from build123d import *

# Parameters (mm, degrees)
F0_R     = 4
F1_DEPTH = 3
F0_R_2   = 11
F2_DEPTH = 1


with BuildPart() as f1:
    # F0 (on Top) → F1 (new body, symmetric)
    with BuildSketch(Plane.XY):
        Circle(F0_R)
        with BuildLine():
            ThreePointArc((-2.304886, -1.5), (-2.75, 0), (-2.304886, 1.5))
            Line((-2.304886, 1.5), (2.304886, 1.5))
            ThreePointArc((2.304886, 1.5), (2.75, 0), (2.304886, -1.5))
            Line((2.304886, -1.5), (-2.304886, -1.5))
        make_face(mode=Mode.SUBTRACT)
    extrude(amount=F1_DEPTH, both=True)

    # F0 (on Top) → F2 (join, symmetric)
    with BuildSketch(Plane.XY):
        Circle(F0_R_2)
        with BuildLine():
            Line((-7.071068, -7.071068), (-4.242641, -4.242641))
            ThreePointArc((-4.242641, -4.242641), (-3.80636, -4.638063), (-3.333421, -4.988818))
            Line((-3.333421, -4.988818), (-5.555702, -8.314696))
            ThreePointArc((-5.555702, -8.314696), (-6.343933, -7.730105), (-7.071068, -7.071068))
        make_face(mode=Mode.SUBTRACT)
        with BuildLine():
            Line((-3.826834, -9.238795), (-2.296101, -5.543277))
            ThreePointArc((-2.296101, -5.543277), (-1.741708, -5.741642), (-1.170542, -5.884712))
            Line((-1.170542, -5.884712), (-1.950903, -9.807853))
            ThreePointArc((-1.950903, -9.807853), (-2.902847, -9.569403), (-3.826834, -9.238795))
        make_face(mode=Mode.SUBTRACT)
        with BuildLine():
            Line((-9.238795, -3.826834), (-5.543277, -2.296101))
            ThreePointArc((-5.543277, -2.296101), (-5.291528, -2.82838), (-4.988818, -3.333421))
            Line((-4.988818, -3.333421), (-8.314696, -5.555702))
            ThreePointArc((-8.314696, -5.555702), (-8.819213, -4.713967), (-9.238795, -3.826834))
        make_face(mode=Mode.SUBTRACT)
        with BuildLine():
            Line((-10, 0), (-6, 0))
            ThreePointArc((-6, 0), (-5.971108, -0.588103), (-5.884712, -1.170542))
            Line((-5.884712, -1.170542), (-9.807853, -1.950903))
            ThreePointArc((-9.807853, -1.950903), (-9.951847, -0.980171), (-10, 0))
        make_face(mode=Mode.SUBTRACT)
        with BuildLine():
            ThreePointArc((1.950903, -9.807853), (0.980171, -9.951847), (0, -10))
            Line((0, -10), (0, -6))
            ThreePointArc((0, -6), (0.588103, -5.971108), (1.170542, -5.884712))
            Line((1.170542, -5.884712), (1.950903, -9.807853))
        make_face(mode=Mode.SUBTRACT)
        with BuildLine():
            Line((3.826834, -9.238795), (2.296101, -5.543277))
            ThreePointArc((2.296101, -5.543277), (2.82838, -5.291528), (3.333421, -4.988818))
            Line((3.333421, -4.988818), (5.555702, -8.314696))
            ThreePointArc((5.555702, -8.314696), (4.713967, -8.819213), (3.826834, -9.238795))
        make_face(mode=Mode.SUBTRACT)
        with BuildLine():
            Line((7.071068, -7.071068), (4.242641, -4.242641))
            ThreePointArc((4.242641, -4.242641), (4.638063, -3.80636), (4.988818, -3.333421))
            Line((4.988818, -3.333421), (8.314696, -5.555702))
            ThreePointArc((8.314696, -5.555702), (7.730105, -6.343933), (7.071068, -7.071068))
        make_face(mode=Mode.SUBTRACT)
        with BuildLine():
            Line((9.238795, -3.826834), (5.543277, -2.296101))
            ThreePointArc((5.543277, -2.296101), (5.741642, -1.741708), (5.884712, -1.170542))
            Line((5.884712, -1.170542), (9.807853, -1.950903))
            ThreePointArc((9.807853, -1.950903), (9.569403, -2.902847), (9.238795, -3.826834))
        make_face(mode=Mode.SUBTRACT)
        with BuildLine():
            Line((-9.238795, 3.826834), (-5.543277, 2.296101))
            ThreePointArc((-5.543277, 2.296101), (-5.741642, 1.741708), (-5.884712, 1.170542))
            Line((-5.884712, 1.170542), (-9.807853, 1.950903))
            ThreePointArc((-9.807853, 1.950903), (-9.569403, 2.902847), (-9.238795, 3.826834))
        make_face(mode=Mode.SUBTRACT)
        with BuildLine():
            Line((-7.071068, 7.071068), (-4.242641, 4.242641))
            ThreePointArc((-4.242641, 4.242641), (-4.638063, 3.80636), (-4.988818, 3.333421))
            Line((-4.988818, 3.333421), (-8.314696, 5.555702))
            ThreePointArc((-8.314696, 5.555702), (-7.730105, 6.343933), (-7.071068, 7.071068))
        make_face(mode=Mode.SUBTRACT)
        with BuildLine():
            Line((-3.826834, 9.238795), (-2.296101, 5.543277))
            ThreePointArc((-2.296101, 5.543277), (-2.82838, 5.291528), (-3.333421, 4.988818))
            Line((-3.333421, 4.988818), (-5.555702, 8.314696))
            ThreePointArc((-5.555702, 8.314696), (-4.713967, 8.819213), (-3.826834, 9.238795))
        make_face(mode=Mode.SUBTRACT)
        with BuildLine():
            Line((0, 10), (0, 6))
            ThreePointArc((0, 6), (-0.588103, 5.971108), (-1.170542, 5.884712))
            Line((-1.170542, 5.884712), (-1.950903, 9.807853))
            ThreePointArc((-1.950903, 9.807853), (-0.980171, 9.951847), (0, 10))
        make_face(mode=Mode.SUBTRACT)
        Circle(F0_R, mode=Mode.SUBTRACT)
        with BuildLine():
            Line((10, 0), (6, 0))
            ThreePointArc((6, 0), (5.971108, 0.588103), (5.884712, 1.170542))
            Line((5.884712, 1.170542), (9.807853, 1.950903))
            ThreePointArc((9.807853, 1.950903), (9.951847, 0.980171), (10, 0))
        make_face(mode=Mode.SUBTRACT)
        with BuildLine():
            Line((9.238795, 3.826834), (5.543277, 2.296101))
            ThreePointArc((5.543277, 2.296101), (5.291528, 2.82838), (4.988818, 3.333421))
            Line((4.988818, 3.333421), (8.314696, 5.555702))
            ThreePointArc((8.314696, 5.555702), (8.819213, 4.713967), (9.238795, 3.826834))
        make_face(mode=Mode.SUBTRACT)
        with BuildLine():
            Line((3.826834, 9.238795), (2.296101, 5.543277))
            ThreePointArc((2.296101, 5.543277), (1.741708, 5.741642), (1.170542, 5.884712))
            Line((1.170542, 5.884712), (1.950903, 9.807853))
            ThreePointArc((1.950903, 9.807853), (2.902847, 9.569403), (3.826834, 9.238795))
        make_face(mode=Mode.SUBTRACT)
        with BuildLine():
            Line((7.071068, 7.071068), (4.242641, 4.242641))
            ThreePointArc((4.242641, 4.242641), (3.80636, 4.638063), (3.333421, 4.988818))
            Line((3.333421, 4.988818), (5.555702, 8.314696))
            ThreePointArc((5.555702, 8.314696), (6.343933, 7.730105), (7.071068, 7.071068))
        make_face(mode=Mode.SUBTRACT)
    extrude(amount=F2_DEPTH, both=True)


solid = f1.part
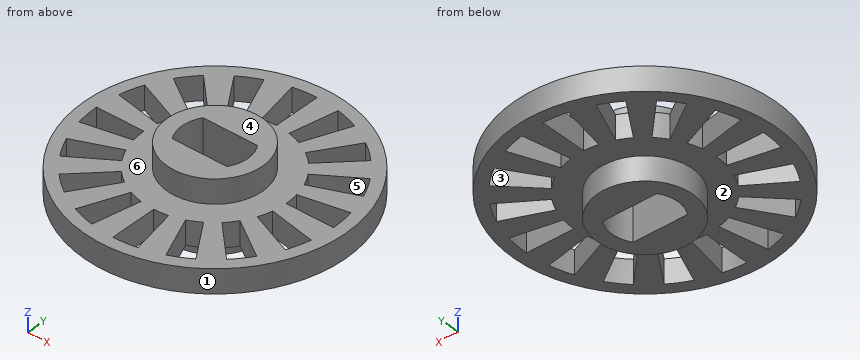
Read the model definition and answer for the solid it produces. Units are mm, in the model's axes. Face numbers are marked on the shaded views. A direction names the side the tool comes from. Coordinates: 2 decimals unless noted, no trailing zeros. Order: outer loops, then holes, each group sorted by start corner. A loop starts at its lowest first (then second) coordinate and runs counter-clockwise, first axis right, second up. Notation, with made-up numbers: (83.5, 42) - (121.5, 42) arc R28 cw to (121.5, 65) - close; hole circle Ø2 at (-40, 74). An arc over 180 degrees is marked (long way). Use one line per item in the form item = value.
(1) Straight lines are drawn through the part: L1, parallel to Y at x = 4.5, z = 0.45; L2, parallel to X at y = 7.5, z = -0.1; L3, parallel to Z at x = -5.5, y = 7.25. For each, find the intervals that lie inside material, in ascending order.
Computed values:
L1 = -10.04 to -8.93, -6.73 to -4.5, -3.97 to 4.5, 6.73 to 10.04
L2 = -8.05 to -5.01, -3.11 to -1.49, 0 to 1.49, 3.11 to 5.01, 6.61 to 8.05
L3 = -1 to 1
(2) Section D-D, the plane x = 8 is taken. Give the vertices of the cut face in (y, z), then the cut area to 3 significant figures.
Computed values:
outline = (-7.55, -1) - (-6, -1) - (-6, 1) - (-7.55, 1) - close; (-5.35, -1) - (-3.31, -1) - (-3.31, 1) - (-5.35, 1) - close; (-1.59, -1) - (0, -1) - (0, 1) - (-1.59, 1) - close; (1.59, -1) - (3.31, -1) - (3.31, 1) - (1.59, 1) - close; (5.35, -1) - (7.55, -1) - (7.55, 1) - (5.35, 1) - close
area = 18.2 mm²
(3) Section C-C, the plane x = -9.5 is taken. Give the vertices of the cut face in (y, z).
Computed values:
outline = (-5.55, -1) - (-1.89, -1) - (-1.89, 1) - (-5.55, 1) - close; (0, -1) - (1.89, -1) - (1.89, 1) - (0, 1) - close; (3.12, -1) - (5.55, -1) - (5.55, 1) - (3.12, 1) - close
(4) Given pin 1 Ø5 at (x, y) = (-3, -7.5) entering from +Z; pin 2 Ø0.6 at (y, z) = (-8, 0) entering from +X; pin 3 Ø1.5 at (x, z) = (-2.5, 1) entering from +Y, each flat-ended and moving along its own axis, determine where each tip first touches the part or whether it passes through.
Computed values:
pin_1 = 1
pin_2 = 7.86
pin_3 = 10.86
(5) For a pull along X with two mould halves and no side action, classify the marked faces 1, 2 and 3 as pulls with the +X half, pulls with the -X half, needs draft (parallel to the pull), parting line crosses it, or undercut.
Computed values:
face_1 = parting line crosses it
face_2 = needs draft
face_3 = undercut
(6) Which of the six approach directions +Z, -Z, +X, -X, +Y, -Y give full straight-line access (tool end or side, diameter ignored) to the marked faces 4, 5 and 6?
Computed values:
face_4 = +Z, +X, -X, +Y, -Y
face_5 = +Z, -Z
face_6 = +Z
(7) Section B-B, the plane z = 1.65 is taken. Give the vertices of the cut face in (x, y).
Computed values:
outline = circle Ø8 at (0, 0); hole (-2.3, -1.5) - (2.3, -1.5) arc R2.75 ccw to (2.3, 1.5) - (-2.3, 1.5) arc R2.75 ccw to start
(8) Section A-A, the plane y = 7.5 is taken. Give the vertices of the cut face in (x, z), then the cut area to 3 significant figures.
Computed values:
outline = (-8.05, -1) - (-5.01, -1) - (-5.01, 1) - (-8.05, 1) - close; (-3.11, -1) - (-1.49, -1) - (-1.49, 1) - (-3.11, 1) - close; (0, -1) - (1.49, -1) - (1.49, 1) - (0, 1) - close; (3.11, -1) - (5.01, -1) - (5.01, 1) - (3.11, 1) - close; (6.61, -1) - (8.05, -1) - (8.05, 1) - (6.61, 1) - close
area = 19.0 mm²
